Source: CAD feature listing. Evaluate the final solid. Frame: model axes, mm. A direction names the side the tool comes from. Give positions to 0.01 mm unless a question says otherwise; leave off trailing zeros. Loops run counter-clockwise (first coordinate to the right, second up) from the corner with the lowest first, then second, coordinate; pieces in that order, holes last. Notation, with made-up numbers: (10.5, -34.5) - (31.5, -34.5) arc R8 ccw to (31.5, -20.5) - close; hole circle Ø4 at (39.25, 63.25). An arc over 180 degrees is marked (long way). Write each question's results on one line, items separated by ' | '. Start each with the question number.
(1) Reachability of faces 5 (the flat face through (-41, -28, 26.068)), 6 (the cylindrical face through (-52.343, -7.605, 51.222)), 7 (the flat face through (-23, -3, -28.652)) from +Z, -Z, +X, -X, +Y, -Y: full face, straight path, thin tool, end or side. Return the list, or none.
(2) Cut plane A-A on y = -92. Return the cut outline in (x, z), then the cut area to 3 significant figures.
(3) Cut plane C-C on z = 11. Return the cut outline in (x, y), then the cut area to 3 significant figures.
(4) Pull-direction query (Y, two-part tool) for faces 1 (the flat face through (-23, -28, 36.068)), 2 (the flat face through (-63.185, -9, 0)), 3 (the flat face through (-24, 0, -44)), 4 (the flat face through (-23.07, -45.27, -13.79)); classes: pulls with the +Y half, pulls with the -Y half, needs draft (parallel to the pull), parting line crosses it, or undercut.
(5) Cut plane B-B on x = -15.5. Return the cut outline in (y, z), then the cut area to 3 significant figures.
(6) Contact query for flat-ended pins moving along their axis: pin 1 (9 mm diameter, centred on x = -48.62, z = 47.81, fed in from -Y); pin 2 (1 mm diameter, centred on x = -17, y = -12.5, fed in from +Z); pin 3 (12 mm diameter, centred on x = -15, z = -44, fed in from -Y). Output: stop coordinate, or through.
(7) Material intervals for line 1 along Y through (x, z) = (-23.5, 44.5); line 2 along Y through (x, z) = (-54.5, 8); line 3 along Y through (x, z) = (-38.5, 18.5), sorted ascending. Write a range as [from, to].
(8) Cut plane D-D on y = -22. Return the cut outline in (x, z), then the cut area to 3 significant figures.
from build123d import *

# Parameters (mm, degrees)
F0_W      = 80
F0_H      = 120
F1_DEPTH  = 15
F3_DEPTH  = 60
F4_R      = 35
F4_R_2    = 25
F5_DEPTH  = 60
F6_R      = 25
F7_DEPTH  = 72.2
F8_W      = 10
F8_H      = 50
F9_DEPTH  = 59.7
F11_DEPTH = 25
F12_R     = 5.047849
F12_R_2   = 5
F13_DEPTH = 39.5
F14_W     = 5
F14_H     = 60
F15_DEPTH = 85.5
F16_R     = 25
F17_DEPTH = 91.3


with BuildPart() as f1:
    # F0 (on Front) → F1 (new body)
    with BuildSketch(Plane.XZ):
        with Locations((-23.184717, 1.068225)):
            Rectangle(F0_W, F0_H)
    extrude(amount=F1_DEPTH)

    # F2 (on face) → F3 (join)
    with BuildSketch(Plane.XZ.offset(15)):
        Polygon((6.815283, 36.068225), (-53.184717, 36.068225), (-53.184717, 26.068225), (-27.741479, 26.068225), (-17.741479, 26.068225), (6.815283, 26.068225), align=None)
    extrude(amount=F3_DEPTH)

    # F4 (on face) → F5 (join)
    with BuildSketch(Plane.YZ.offset(6.815283)):
        with Locations((-75, 31.068225)):
            Circle(F4_R)
        with Locations((-75, 31.068225)):
            Circle(F4_R_2, mode=Mode.SUBTRACT)
    extrude(amount=-F5_DEPTH)

    # F6 (on face) → F7 (cut)
    with BuildSketch(Plane.YZ.offset(6.815283)):
        with Locations((-75, 31.068225)):
            Circle(F6_R)
    extrude(amount=-F7_DEPTH, mode=Mode.SUBTRACT)

    # F8 (on face) → F9 (join)
    with BuildSketch(Plane.XZ.offset(15)):
        with Locations((-23.003544, 1.068225)):
            Rectangle(F8_W, F8_H)
    extrude(amount=F9_DEPTH)

    # F10 (on face) → F11 (cut)
    with BuildSketch(Plane(origin=(-28.003544, 0, 0), x_dir=(0, -1, 0), z_dir=(-1, 0, 0))):
        Polygon((87.144889, -23.931775), (74.7, -3.930489), (15, -23.931775), (56.138653, -39.033107), align=None)
    extrude(amount=-F11_DEPTH, mode=Mode.SUBTRACT)

    # F12 (on face) → F13 (cut)
    with BuildSketch(Plane.XZ.offset(15)):
        with Locations((-48.622161, -45.490056)):
            Circle(F12_R)
        with Locations((1.377839, -45.490056)):
            Circle(F12_R_2)
        with Locations((-48.622161, 47.809944)):
            Circle(F12_R)
        with Locations((1.377839, 47.809944)):
            Circle(F12_R_2)
    extrude(amount=-F13_DEPTH, mode=Mode.SUBTRACT)

    # F14 (on face) → F15 (cut)
    with BuildSketch(Plane.YZ.offset(16.815283)):
        with Locations((-2.5, 1.347677)):
            Rectangle(F14_W, F14_H)
    extrude(amount=-F15_DEPTH, mode=Mode.SUBTRACT)

    # F16 (on face) → F17 (cut)
    with BuildSketch(Plane(origin=(-53.184717, 0, 0), x_dir=(0, -1, 0), z_dir=(-1, 0, 0))):
        with Locations((75, 31.068225)):
            Circle(F16_R)
    extrude(amount=-F17_DEPTH, mode=Mode.SUBTRACT)


solid = f1.part
Ans:
1) face 5: -Z, -X | face 6: +Y | face 7: +X, -X, +Y
2) outline: (-53.18, 0.47) - (6.82, 0.47) - (6.82, 12.74) - (-53.18, 12.74) - close; (-53.18, 49.4) - (6.82, 49.4) - (6.82, 61.66) - (-53.18, 61.66) - close | area: 1,470 mm^2
3) outline: (-63.18, -15) - (-28, -15) - (-28, -46.32) - (-53.18, -46.32) - (-53.18, -60.09) - (6.82, -60.09) - (6.82, -46.32) - (-18, -46.32) - (-18, -15) - (16.82, -15) - (16.82, -5) - (-63.18, -5) - close; (-53.18, -103.68) - (6.82, -103.68) - (6.82, -89.91) - (-53.18, -89.91) - close | area: 2,770 mm^2
4) face 1: undercut | face 2: needs draft | face 3: pulls with the +Y half | face 4: pulls with the -Y half
5) outline: (-40.36, 26.07) - (-15, 26.07) - (-15, -58.93) - (0, -58.93) - (0, -28.65) - (-5, -28.65) - (-5, 31.35) - (0, 31.35) - (0, 61.07) - (-15, 61.07) - (-15, 36.07) - (-40.36, 36.07) arc R35 ccw (long way) to start; hole circle Ø50 at (-75, 31.07) | area: 3,640 mm^2
6) pin 1: y = -107.79 | pin 2: z = 61.07 | pin 3: y = -15
7) line 1: [-107.32, -96.09], [-53.91, -42.68], [-15, 0] | line 2: [-15, -5] | line 3: [-107.67, -96.61], [-53.39, -42.33], [-15, -5]
8) outline: (-53.18, 26.07) - (-28, 26.07) - (-28, -21.59) - (-18, -21.59) - (-18, 26.07) - (6.82, 26.07) - (6.82, 36.07) - (-53.18, 36.07) - close | area: 1,080 mm^2
